```python
from build123d import *

# Parameters (mm, degrees)
SKETCH1_W              = 65.5
SKETCH1_H              = 9
SKETCH1_R              = 0.998395378
SKETCH1_R_2            = 1.243115981
BOSS_EXTRUDE1_DEPTH    = 6
SKETCH3_W              = 65.5
SKETCH3_H              = 6
BOSS_EXTRUDE2_DEPTH    = 10
SKETCH4_W              = 65.5
SKETCH4_H              = 6
BOSS_EXTRUDE3_DEPTH    = 2
SKETCH5_W              = 65.5
SKETCH5_H              = 3
BOSS_EXTRUDE4_DEPTH    = 9.2
SKETCH7_W              = 21
SKETCH7_H              = 15.2
BOSS_EXTRUDE6_DEPTH    = 3
SKETCH12_W             = 68.5
SKETCH12_H             = 15.2
BOSS_EXTRUDE10_DEPTH   = 3
SKETCH13_W             = 24
SKETCH13_H             = 15.2
SKETCH13_W_2           = 12
SKETCH13_H_2           = 3.7
BOSS_EXTRUDE11_DEPTH   = 3
CUT_EXTRUDE2_DEPTH     = 46.662922596
SKETCH11_W             = 18
SKETCH11_H             = 9.2
CUT_EXTRUDE4_DEPTH     = 3
SKETCH14_W             = 71.5
SKETCH14_H             = 24
BOSS_EXTRUDE12_DEPTH   = 3
SKETCH15_W             = 65.5
SKETCH15_H             = 3.5
CUT_EXTRUDE5_DEPTH     = 3
SKETCH16_R             = 3
CUT_EXTRUDE6_DEPTH     = 15.2
MIRROR10_OUTLINE_W     = 71.5
MIRROR10_OUTLINE_H     = 24
MIRROR10_OUTLINE_R     = 3
MIRROR10_DEPTH         = 6
MIRROR10_START         = 6
MIRROR10_2_DEPTH       = 12.2
MIRROR10_START_2       = 15.2
MIRROR10_3_OUTLINE_W   = 65.5
MIRROR10_3_OUTLINE_H   = 3.5
MIRROR10_3_OUTLINE_R   = 3
MIRROR10_3_DEPTH       = 3
MIRROR10_4_OUTLINE_R   = 3
MIRROR10_4_OUTLINE_R_2 = 1.243115981
MIRROR10_4_OUTLINE_R_3 = 0.998395378
MIRROR10_4_DEPTH       = 3
MIRROR10_5_OUTLINE_W   = 3
MIRROR10_5_OUTLINE_H   = 12
MIRROR10_5_DEPTH       = 2.75
MIRROR10_START_3       = 12.45
MIRROR10_6_OUTLINE_W   = 3
MIRROR10_6_OUTLINE_H   = 12
MIRROR10_6_DEPTH       = 2.75
MIRROR10_START_4       = -17.5
MIRROR10_7_DEPTH       = 24
SKETCH17_W             = 71.5
SKETCH17_H             = 24
CUT_EXTRUDE7_DEPTH     = 111.181906409


with BuildPart() as part:
    # Sketch1 → Boss-Extrude1 (new body)
    with BuildSketch(Plane(origin=(0, 0, 0), x_dir=(1, 0, 0), z_dir=(0, 1, 0))):
        Rectangle(SKETCH1_W, SKETCH1_H)
        with Locations(Location((-29.75, 0, 0), (0, 0, 270))):
            Circle(SKETCH1_R, mode=Mode.SUBTRACT)
        with Locations(Location((29.75, 0, 0), (0, 0, 270))):
            Circle(SKETCH1_R_2, mode=Mode.SUBTRACT)
    extrude(amount=BOSS_EXTRUDE1_DEPTH)

    # Sketch3 → Boss-Extrude2 (add)
    with BuildSketch(Plane(origin=(0, 0, -4.5), x_dir=(-1, 0, 0), z_dir=(0, 0, -1))):
        with Locations((0, 3)):
            Rectangle(SKETCH3_W, SKETCH3_H)
    extrude(amount=BOSS_EXTRUDE2_DEPTH)

    # Sketch4 → Boss-Extrude3 (add)
    with BuildSketch(Plane.XY.offset(4.5)):
        with Locations((0, 3)):
            Rectangle(SKETCH4_W, SKETCH4_H)
    extrude(amount=BOSS_EXTRUDE3_DEPTH)

    # Sketch5 → Boss-Extrude4 (add)
    with BuildSketch(Plane(origin=(0, 6, 0), x_dir=(1, 0, 0), z_dir=(0, 1, 0))):
        with Locations((0, -5)):
            Rectangle(SKETCH5_W, SKETCH5_H)
    extrude(amount=BOSS_EXTRUDE4_DEPTH)

    # Sketch7 → Boss-Extrude6 (add)
    with BuildSketch(Plane.ZY.offset(32.75)):
        with Locations((-4, 7.6)):
            Rectangle(SKETCH7_W, SKETCH7_H)
    extrude(amount=BOSS_EXTRUDE6_DEPTH)

    # Sketch12 → Boss-Extrude10 (add)
    with BuildSketch(Plane(origin=(0, 0, -14.5), x_dir=(-1, 0, 0), z_dir=(0, 0, -1))):
        with Locations((1.5, 7.6)):
            Rectangle(SKETCH12_W, SKETCH12_H)
    extrude(amount=BOSS_EXTRUDE10_DEPTH)

    # Sketch13 → Boss-Extrude11 (add)
    with BuildSketch(Plane(origin=(32.75, 0, 0), x_dir=(0, 0, -1), z_dir=(1, 0, 0))):
        with Locations((5.5, 7.6)):
            Rectangle(SKETCH13_W, SKETCH13_H)
        with Locations((5.5, 10.6)):
            Rectangle(SKETCH13_W_2, SKETCH13_H_2, mode=Mode.SUBTRACT)
    extrude(amount=BOSS_EXTRUDE11_DEPTH)

    # Sketch6 → Cut-Extrude2 (cut, through all)
    with BuildSketch(Plane.XY.offset(6.5)):
        with BuildLine():
            ThreePointArc((-23.75, 10.6), (-24.628679656, 12.721320344), (-26.75, 13.6))
            Line((-26.75, 13.6), (-26.75, 7.6))
            ThreePointArc((-26.75, 7.6), (-24.628679656, 8.478679656), (-23.75, 10.6))
        make_face()
        with BuildLine():
            Line((-26.75, 7.6), (-26.75, 13.6))
            ThreePointArc((-26.75, 13.6), (-29.75, 10.6), (-26.75, 7.6))
        make_face()
        with BuildLine():
            ThreePointArc((29.75, 10.6), (28.871320344, 12.721320344), (26.75, 13.6))
            Line((26.75, 13.6), (26.75, 7.6))
            ThreePointArc((26.75, 7.6), (28.871320344, 8.478679656), (29.75, 10.6))
        make_face()
        with BuildLine():
            Line((26.75, 7.6), (26.75, 13.6))
            ThreePointArc((26.75, 13.6), (23.75, 10.6), (26.75, 7.6))
        make_face()
        with BuildLine():
            Line((26.75, 13.6), (-26.75, 13.6))
            ThreePointArc((-26.75, 13.6), (-24.628679656, 12.721320344), (-23.75, 10.6))
            ThreePointArc((-23.75, 10.6), (-24.628679656, 8.478679656), (-26.75, 7.6))
            Line((-26.75, 7.6), (26.75, 7.6))
            ThreePointArc((26.75, 7.6), (23.75, 10.6), (26.75, 13.6))
        make_face()
    extrude(amount=-CUT_EXTRUDE2_DEPTH, mode=Mode.SUBTRACT)

    # Sketch11 → Cut-Extrude4 (cut)
    with BuildSketch(Plane.ZY.offset(35.75)):
        with Locations((-5.5, 10.6)):
            Rectangle(SKETCH11_W, SKETCH11_H)
    extrude(amount=-CUT_EXTRUDE4_DEPTH, mode=Mode.SUBTRACT)

    # Sketch14 → Boss-Extrude12 (add)
    with BuildSketch(Plane(origin=(0, 15.2, 0), x_dir=(1, 0, 0), z_dir=(0, 1, 0))):
        with Locations((0, 5.5)):
            Rectangle(SKETCH14_W, SKETCH14_H)
    extrude(amount=BOSS_EXTRUDE12_DEPTH)

    # Sketch15 → Cut-Extrude5 (cut)
    with BuildSketch(Plane(origin=(0, 18.2, 0), x_dir=(1, 0, 0), z_dir=(0, 1, 0))):
        with Locations((0, 5.5)):
            Rectangle(SKETCH15_W, SKETCH15_H)
    extrude(amount=-CUT_EXTRUDE5_DEPTH, mode=Mode.SUBTRACT)

    # Sketch16 → Cut-Extrude6 (cut)
    with BuildSketch(Plane(origin=(0, 18.2, 0), x_dir=(1, 0, 0), z_dir=(0, 1, 0))):
        with Locations(Location((-29.75, 0, 0), (0, 0, 270))):
            Circle(SKETCH16_R)
        with Locations(Location((29.75, 0, 0), (0, 0, 270))):
            Circle(SKETCH16_R)
    extrude(amount=-CUT_EXTRUDE6_DEPTH, mode=Mode.SUBTRACT)

    # Mirror10: read off the stored shape, not the designer's step
    # Mirror10 outline → Mirror10 (add)
    with BuildSketch(Plane(origin=(0, 0, 0), x_dir=(1, 0, 0), z_dir=(0, 1, 0))):
        with Locations((71.5, 5.5)):
            Rectangle(MIRROR10_OUTLINE_W, MIRROR10_OUTLINE_H)
        with Locations((41.75, 0)):
            Circle(MIRROR10_OUTLINE_R, mode=Mode.SUBTRACT)
        with Locations((101.25, 0)):
            Circle(MIRROR10_OUTLINE_R, mode=Mode.SUBTRACT)
    extrude(amount=MIRROR10_DEPTH)

    # Mirror10 2 outline → Mirror10 2 (add)
    with BuildSketch(Plane(origin=(0, 0, 0), x_dir=(1, 0, 0), z_dir=(0, 1, 0)).offset(MIRROR10_START)):
        Polygon((35.75, -0.5), (35.75, -6.5), (107.25, -6.5), (107.25, -3.5), (38.75, -3.5), (38.75, -0.5), align=None)
        Polygon((35.75, 17.5), (35.75, 11.5), (38.75, 11.5), (38.75, 14.5), (107.25, 14.5), (107.25, 17.5), align=None)
    extrude(amount=MIRROR10_2_DEPTH)

    # Mirror10 3 outline → Mirror10 3 (add)
    with BuildSketch(Plane(origin=(0, 0, 0), x_dir=(1, 0, 0), z_dir=(0, 1, 0)).offset(MIRROR10_START_2)):
        Polygon((35.75, 11.5), (35.75, -0.5), (38.75, -0.5), (38.75, -3.5), (107.25, -3.5), (107.25, 14.5), (38.75, 14.5), (38.75, 11.5), align=None)
        with Locations((71.5, 5.5)):
            Rectangle(MIRROR10_3_OUTLINE_W, MIRROR10_3_OUTLINE_H, mode=Mode.SUBTRACT)
        with Locations((41.75, 0)):
            Circle(MIRROR10_3_OUTLINE_R, mode=Mode.SUBTRACT)
        with Locations((101.25, 0)):
            Circle(MIRROR10_3_OUTLINE_R, mode=Mode.SUBTRACT)
    extrude(amount=MIRROR10_3_DEPTH)

    # Mirror10 4 outline → Mirror10 4 (add)
    # profile 1 of 2: a face of its own
    with BuildSketch(Plane(origin=(0, 0, 0), x_dir=(1, 0, 0), z_dir=(0, 1, 0))):
        with Locations((41.75, 0)):
            Circle(MIRROR10_4_OUTLINE_R)
        with Locations((41.75, 0)):
            Circle(MIRROR10_4_OUTLINE_R_2, mode=Mode.SUBTRACT)
    # profile 2 of 2: a face of its own
    with BuildSketch(Plane(origin=(0, 0, 0), x_dir=(1, 0, 0), z_dir=(0, 1, 0))):
        with Locations((101.25, 0)):
            Circle(MIRROR10_4_OUTLINE_R)
        with Locations((101.25, 0)):
            Circle(MIRROR10_4_OUTLINE_R_3, mode=Mode.SUBTRACT)
    extrude(amount=MIRROR10_4_DEPTH)

    # Mirror10 5 outline → Mirror10 5 (add)
    with BuildSketch(Plane(origin=(0, 0, 0), x_dir=(1, 0, 0), z_dir=(0, 1, 0)).offset(MIRROR10_START)):
        with Locations((37.25, 5.5)):
            Rectangle(MIRROR10_5_OUTLINE_W, MIRROR10_5_OUTLINE_H)
    extrude(amount=MIRROR10_5_DEPTH)

    # Mirror10 6 outline → Mirror10 6 (add)
    with BuildSketch(Plane(origin=(0, 0, 0), x_dir=(1, 0, 0), z_dir=(0, 1, 0)).offset(MIRROR10_START_3)):
        with Locations((37.25, 5.5)):
            Rectangle(MIRROR10_6_OUTLINE_W, MIRROR10_6_OUTLINE_H)
    extrude(amount=MIRROR10_6_DEPTH)

    # Mirror10 7 outline → Mirror10 7 (cut)
    with BuildSketch(Plane.XY.offset(MIRROR10_START_4)):
        with BuildLine():
            Line((44.75, 7.6), (98.25, 7.6))
            ThreePointArc((98.25, 7.6), (101.25, 10.6), (98.25, 13.6))
            Line((98.25, 13.6), (44.75, 13.6))
            ThreePointArc((44.75, 13.6), (41.75, 10.6), (44.75, 7.6))
        make_face()
    extrude(amount=MIRROR10_7_DEPTH, mode=Mode.SUBTRACT)

    # Sketch17 → Cut-Extrude7 (cut, through all)
    with BuildSketch(Plane(origin=(0, 18.2, 0), x_dir=(1, 0, 0), z_dir=(0, 1, 0))):
        with Locations((0, 5.5)):
            Rectangle(SKETCH17_W, SKETCH17_H)
    extrude(amount=-CUT_EXTRUDE7_DEPTH, mode=Mode.SUBTRACT)


solid = part.part
```
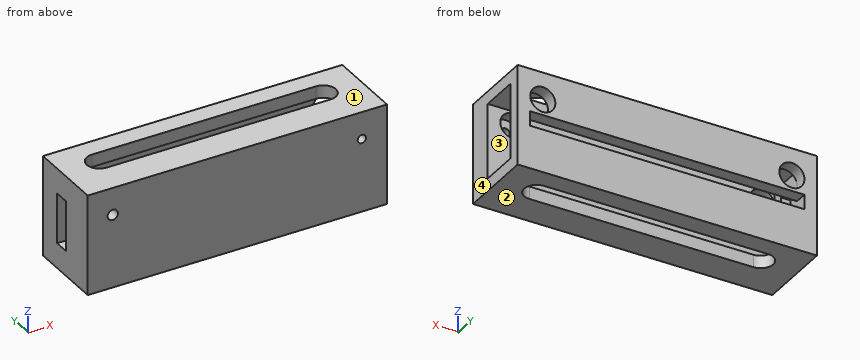
Check sheet for the modelled part. Datum: model origin and axes. Units: mm. Face numbers are marked on the shaded views. Round coordinates to 2 decimals unless told otherwise and drop trailing zeros. Order: outer loops, then holes, each group sorted by start corner. A loop starts at its lowest first (then second) coordinate and runs counter-clockwise, first axis right, second up.
1) Section check B-B (x = 86). Record the boundary of the cut face in (y, z).
2) Section check D-D (y = 9.5). Record the boundary of the cut face in (x, z).
3) Go/stop test with a flat-tipped pin: pin 1 Ø3.5 at (x, z) = (41.75, 0) entering from +Y. Record where the tip stops, or that it passes through.
4) Scan lines: line 1 (X direction, y = 15.95, z = 0); line 2 (Z direction, x = 101.25, y = 16.6); line 3 (Z direction, x = 99.5, y = 7). Record each from-to range of solid material in increasing order.
5) Mould release check, pull along Z, two halves, no side actions. Record for the marked faces 1, 2, 3 and 4: +Z half, -Z half, draft (parallel to the pull), parting line (faces both ways), or undercut.
6) Section check C-C (y = 14.25). Record the boundary of the cut face in (x, z).
7) Section check A-A (z = -8). Record the boundary of the cut face in (x, y), and give its area (3 significant figures).
Result:
1. outline: (0, -17.5) - (7.6, -17.5) - (7.6, -14.5) - (6, -14.5) - (6, 3.5) - (7.6, 3.5) - (7.6, 6.5) - (0, 6.5) - close; (13.6, -17.5) - (18.2, -17.5) - (18.2, -7.25) - (15.2, -7.25) - (15.2, -14.5) - (13.6, -14.5) - close; (13.6, 3.5) - (15.2, 3.5) - (15.2, -3.75) - (18.2, -3.75) - (18.2, 6.5) - (13.6, 6.5) - close
2. outline: (35.75, -17.5) - (41.96, -17.5) - (41.96, -14.5) - (38.75, -14.5) - (38.75, -11.5) - (35.75, -11.5) - close; (35.75, 0.5) - (38.75, 0.5) - (38.75, 3.5) - (41.96, 3.5) - (41.96, 6.5) - (35.75, 6.5) - close; (101.04, -17.5) - (107.25, -17.5) - (107.25, -14.5) - (101.04, -14.5) - close; (101.04, 3.5) - (107.25, 3.5) - (107.25, 6.5) - (101.04, 6.5) - close
3. pin 1: stops at y = 3
4. line 1: x = 35.75 to 38.75, 44.75 to 98.25, 104.25 to 107.25
4. line 2: z = -17.5 to -7.25, -3.75 to -3, 3 to 6.5
4. line 3: z = -17.5 to -14.5, 3.5 to 6.5
5. face 1: +Z half
5. face 2: -Z half
5. face 3: undercut
5. face 4: draft
6. outline: (35.75, -17.5) - (107.25, -17.5) - (107.25, -14.5) - (38.75, -14.5) - (38.75, 3.5) - (107.25, 3.5) - (107.25, 6.5) - (35.75, 6.5) - close
7. outline: (35.75, 0) - (107.25, 0) - (107.25, 6) - (38.75, 6) - (38.75, 8.75) - (35.75, 8.75) - close; (35.75, 12.45) - (38.75, 12.45) - (38.75, 15.2) - (107.25, 15.2) - (107.25, 18.2) - (35.75, 18.2) - close
7. area: 660 mm2
